Verification items for the finished model (mm, model axes). A direction names the side the tool comes from. Give positions to 0.01 mm unless a question says otherwise; leave off trailing zeros. Write each loop counter-clockwise with the first axis right and the second up, starting at its lowest first coordinate (ties: lowest second). Pieces come first, ordered by that corner, then holes. Notation, with made-up numbers: M -8.75,23 L 20.25,23 A3 cw 20.25,27 Z; hole C 54.25,3 d1. An arc over 180 degrees is marked long. Write item = value, one per line.
from build123d import *

# Parameters (mm, degrees)
SKETCH1_W           = 37
SKETCH1_H           = 37
BOSS_EXTRUDE1_DEPTH = 165.35
CUT_EXTRUDE1_DEPTH  = 50
BOSS_EXTRUDE2_START = -10
BOSS_EXTRUDE2_DEPTH = 20
BOSS_EXTRUDE3_START = -40
BOSS_EXTRUDE3_DEPTH = 1.5
CUT_EXTRUDE2_DEPTH  = 10
SKETCH6_R           = 10
CUT_EXTRUDE3_DEPTH  = 10
SKETCH7_R           = 10
CUT_EXTRUDE4_DEPTH  = 10


with BuildPart() as part:
    # Sketch1 → Boss-Extrude1 (new body)
    with BuildSketch(Plane.XY):
        with BuildLine():
            Line((0.305025041, 0), (39.694974959, 0))
            ThreePointArc((39.694974959, 0), (39.910660234, 0.089339766), (40, 0.305025041))
            Line((40, 0.305025041), (40, 39.694974959))
            ThreePointArc((40, 39.694974959), (39.910660234, 39.910660234), (39.694974959, 40))
            Line((39.694974959, 40), (0.305025041, 40))
            ThreePointArc((0.305025041, 40), (0.089339766, 39.910660234), (0, 39.694974959))
            Line((0, 39.694974959), (0, 0.305025041))
            ThreePointArc((0, 0.305025041), (0.089339766, 0.089339766), (0.305025041, 0))
        make_face()
        with Locations((20, 20)):
            Rectangle(SKETCH1_W, SKETCH1_H, mode=Mode.SUBTRACT)
    extrude(amount=BOSS_EXTRUDE1_DEPTH)

    # Sketch2 → Cut-Extrude1 (cut)
    with BuildSketch(Plane(origin=(40, 0, 0), x_dir=(0, 0, -1), z_dir=(1, 0, 0))):
        Polygon((0, 40), (-69.282032303, 0), (0, 0), align=None)
        Polygon((-165.35, 40), (-142.255989232, 0), (-165.35, 0), align=None)
    extrude(amount=-CUT_EXTRUDE1_DEPTH, mode=Mode.SUBTRACT)

    # Sketch3 → Boss-Extrude2 (add)
    with BuildSketch(Plane.ZY.offset(BOSS_EXTRUDE2_START)):
        Polygon((69.282032303, 0), (52.282032303, 0), (52.282032303, 1.5), (66.683956091, 1.5), align=None)
    extrude(amount=-BOSS_EXTRUDE2_DEPTH)

    # Sketch4 → Boss-Extrude3 (add)
    with BuildSketch(Plane.ZY.offset(BOSS_EXTRUDE3_START)):
        Polygon((2.320508076, 30), (19.641016151, 20), (34.641016151, 20), (17.320508076, 30), align=None)
    extrude(amount=BOSS_EXTRUDE3_DEPTH)

    # Sketch5 → Cut-Extrude2 (cut)
    with BuildSketch(Plane(origin=(40, 0, 0), x_dir=(0, 0, -1), z_dir=(1, 0, 0))):
        Polygon((-44.784609691, 28), (-72.497422612, 12), (-138.791887617, 12), (-148.029491924, 28), align=None)
    extrude(amount=-CUT_EXTRUDE2_DEPTH, mode=Mode.SUBTRACT)

    # Sketch6 → Cut-Extrude3 (cut)
    with BuildSketch(Plane(origin=(0, 40, 0), x_dir=(1, 0, 0), z_dir=(0, 1, 0))):
        with Locations(Location((20, -120.35, 0), (0, 0, 180))):
            Circle(SKETCH6_R)
        with Locations(Location((20, -45, 0), (0, 0, 90))):
            Circle(SKETCH6_R)
    extrude(amount=-CUT_EXTRUDE3_DEPTH, mode=Mode.SUBTRACT)

    # Sketch7 → Cut-Extrude4 (cut)
    with BuildSketch(Plane(origin=(1.5, 0, 0), x_dir=(0, 0, -1), z_dir=(1, 0, 0))):
        with Locations((-99.35, 20)):
            Circle(SKETCH7_R)
    extrude(amount=-CUT_EXTRUDE4_DEPTH, mode=Mode.SUBTRACT)


solid = part.part
1) Material ranges on probe 1 along X at (y, z) = (38, 79); probe 2 along X at (y, z) = (39, 120), recorded low to high. Write a range as from..to.
From the geometry:
probe_1 = 0..1.5, 38.5..40
probe_2 = 0..10.01, 29.99..40
2) Draft check along Y on faces 1 (the flat face through (38.5, 32, 82)), 2 (the flat face through (39.26, 19.888, 143.346)), 3 (the flat face through (39.26, 25.07, 10.86)), 4 (the cylindrical face through (20, 39, 55)). Enter one of: +Y half, -Y half, draft (parallel to the pull), parting line (faces both ways), or undercut.
From the geometry:
face_1 = undercut
face_2 = undercut
face_3 = -Y half
face_4 = draft
3) Depth check by flat-ended pin: P1, Ø1.2, axis at x = 22.5, y = 1, coming from the -Z side; P2, Ø18, axis at x = 20, z = 45, coming from the +Y side; P3, Ø1.6, axis at y = 1, z = 59, coming from the +X side. Enter the tip coordinate at first touch or a pass-through.
From the geometry:
P1 = 52.28
P2 = 1.5
P3 = 30
4) Cross-section at C-C on y = 3.5. Record the boundary of the cut face in (x, z).
From the geometry:
outline = M 0,63.22 L 1.5,63.22 L 1.5,144.28 L 0,144.28 Z; M 38.5,63.22 L 40,63.22 L 40,144.28 L 38.5,144.28 Z
5) Tool access check on faces 5 (the flat face through (38.727, 7.084, 57.013)), 6 (the flat face through (39.26, 20.11, 58.45)), 7 (the cylindrical face through (0.76, 26.76, 106.72)), 8 (the cylindrical face through (14.62, 39.26, 128.78)), 9 (the flat face through (1.5, 24, 82)). Record the directions out of +Z, -Z, +X, -X, +Y, -Y that give a thin tool (end or side, any length) a straight path to the whole face; none if there is none.
From the geometry:
face_5 = -Z, +X, -Y
face_6 = +X
face_7 = -X
face_8 = +Y
face_9 = +Z, -Z
6) Cross-section at A-A on z = 99.35. Record the boundary of the cut face in (x, y).
From the geometry:
outline = M 0,0.31 A0.31 ccw 0.31,0 L 39.69,0 A0.31 ccw 40,0.31 L 40,12 L 38.5,12 L 38.5,1.5 L 1.5,1.5 L 1.5,10 L 0,10 Z; M 0,30 L 1.5,30 L 1.5,38.5 L 38.5,38.5 L 38.5,28 L 40,28 L 40,39.69 A0.31 ccw 39.69,40 L 0.31,40 A0.31 ccw 0,39.69 Z
7) Cross-section at B-B on x = 31.5. Record the boundary of the cut face in (y, z).
From the geometry:
outline = M 0,69.28 L 1.5,66.68 L 1.5,143.12 L 0,142.26 Z; M 38.5,2.6 L 40,0 L 40,165.35 L 38.5,164.48 Z
8) Cross-section at D-D on z = 62. Record the boundary of the cut face in (x, y), plus the area to 3 significant figures.
From the geometry:
outline = M 0,4.2 L 1.5,4.2 L 1.5,38.5 L 38.5,38.5 L 38.5,28 L 40,28 L 40,39.69 A0.31 ccw 39.69,40 L 0.31,40 A0.31 ccw 0,39.69 Z; M 10,0 L 30,0 L 30,1.5 L 10,1.5 Z; M 38.5,4.2 L 40,4.2 L 40,18.06 L 38.5,18.06 Z
area = 178 mm^2
